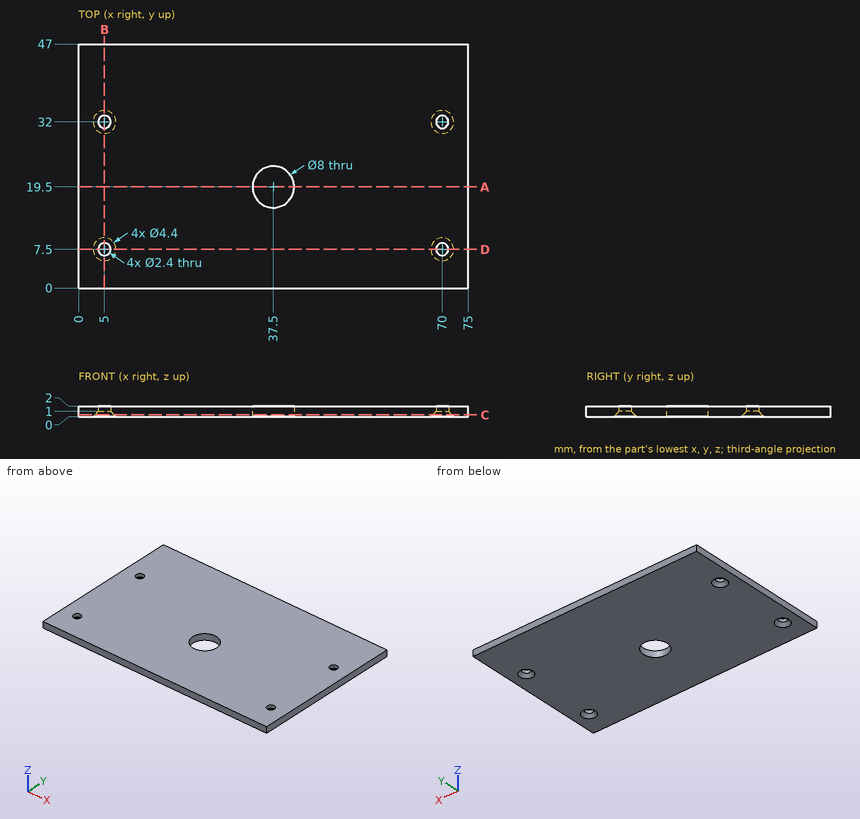
Here's the drawing with two shaded views (mm, measured from the low corner). I have some questions. Round coordinates to 2 decimals unless told otherwise and drop trailing zeros. Order: outer loops, then holes, each group sorted by start corner. A loop starts at its lowest first (then second) coordinate and runs counter-clockwise, first axis right, second up. Notation, with made-up numbers: (59, 33.25) -> (92, 33.25) arc R18 cw to (92, 41.25) -> close; hole circle Ø3 at (10.25, 6). An arc over 180 degrees is marked (long way). Write each question's results on one line, items separated by ' | '. Start each with the question number.
Item 1: If we section it at D-D, the plane y = 7.5: Write out the boundary of the cut face in (x, z).
Item 2: Please list where these lines run through material, in increasing order: L1, parallel to X at y = 7.5, z = 1.6; L2, parallel to Y at x = 70, z = 1.75; L3, parallel to X at y = 31, z = 1.6.
Item 3: Will these pins go through, and if not, where does the flat tip stop? pin 1 (4 mm diameter, centred on x = 51.5, y = 22, fed in from -Z); pin 2 (1.9 mm diameter, centred on x = 5, y = 32, fed in from +Z).
Item 4: If we section it at C-C, the plane z = 0.35: Write out the boundary of the cut face in (x, y), then the cut area to 3 significant figures.
Item 5: If we section it at B-B, the plane x = 5: Write out the boundary of the cut face in (y, z).
Item 6: If we section it at A-A, the plane y = 19.5: Write out the boundary of the cut face in (x, z), then the cut area to 3 significant figures.
Results:
1) outline: (0, 0) -> (2.8, 0) -> (3.8, 1) -> (3.8, 2) -> (0, 2) -> close; (6.2, 1) -> (7.2, 0) -> (67.8, 0) -> (68.8, 1) -> (68.8, 2) -> (6.2, 2) -> close; (71.2, 1) -> (72.2, 0) -> (75, 0) -> (75, 2) -> (71.2, 2) -> close
2) L1: x = 0 to 3.8, 6.2 to 68.8, 71.2 to 75 | L2: y = 0 to 6.3, 8.7 to 30.8, 33.2 to 47 | L3: x = 0 to 4.34, 5.66 to 69.34, 70.66 to 75
3) pin 1: stops at z = 0 | pin 2: passes through
4) outline: (0, 0) -> (75, 0) -> (75, 47) -> (0, 47) -> close; hole circle Ø3.7 at (5, 7.5); hole circle Ø3.7 at (5, 32); hole circle Ø8 at (37.5, 19.5); hole circle Ø3.7 at (70, 7.5); hole circle Ø3.7 at (70, 32) | area: 3,430 mm2
5) outline: (0, 0) -> (5.3, 0) -> (6.3, 1) -> (6.3, 2) -> (0, 2) -> close; (8.7, 1) -> (9.7, 0) -> (29.8, 0) -> (30.8, 1) -> (30.8, 2) -> (8.7, 2) -> close; (33.2, 1) -> (34.2, 0) -> (47, 0) -> (47, 2) -> (33.2, 2) -> close
6) outline: (0, 0) -> (33.5, 0) -> (33.5, 2) -> (0, 2) -> close; (41.5, 0) -> (75, 0) -> (75, 2) -> (41.5, 2) -> close | area: 134 mm2
